from build123d import *

# Parameters (mm, degrees)
SKETCH_1_W      = 20
SKETCH_1_H      = 40
SKETCH_1_R      = 1.8
SKETCH_1_W_2    = 40
SKETCH_1_H_2    = 20
EXTRUDE_1_DEPTH = 3
FILLET_1_R      = 3


with BuildPart() as part:
    # 草图1 → 凸台-拉伸1 (new body)
    # profile 1 of 2: a face of its own
    with BuildSketch(Plane(origin=(0, 0, 0), x_dir=(1, 0, 0), z_dir=(0, 1, 0))):
        with Locations((-10, 30)):
            Rectangle(SKETCH_1_W, SKETCH_1_H)
        with Locations(Location((-10, 20, 0), (0, 0, 270))):
            Circle(SKETCH_1_R, mode=Mode.SUBTRACT)
        with Locations(Location((-10, 40, 0), (0, 0, 270))):
            Circle(SKETCH_1_R, mode=Mode.SUBTRACT)
    # profile 2 of 2: a face of its own
    with BuildSketch(Plane(origin=(0, 0, 0), x_dir=(1, 0, 0), z_dir=(0, 1, 0))):
        Rectangle(SKETCH_1_W_2, SKETCH_1_H_2)
        with Locations(Location((10, 0, 0), (0, 0, 270))):
            Circle(SKETCH_1_R, mode=Mode.SUBTRACT)
        with Locations(Location((-10, 0, 0), (0, 0, 270))):
            Circle(SKETCH_1_R, mode=Mode.SUBTRACT)
    extrude(amount=EXTRUDE_1_DEPTH)

    # 圆角1
    fillet_1_edges = [part.edges().sort_by_distance(p)[0] for p in [
        (-20, 1.5, -50),
        (0, 1.5, -50),
        (20, 1.5, -10),
        (20, 1.5, 10),
        (-20, 1.5, 10),
    ]]
    fillet(fillet_1_edges, radius=FILLET_1_R)


solid = part.part
Verification items for the finished model (mm, model axes). A direction names the side the tool comes from. Coordinates: 2 decimals unless noted, no trailing zeros. Order: outer loops, then holes, each group sorted by start corner. A loop starts at its lowest first (then second) coordinate and runs counter-clockwise, first axis right, second up. Notation, with made-up numbers: (87.5, 60) -> (125.5, 60) arc R22 ccw to (125.5, 70) -> close; hole circle Ø3 at (25, 20). An arc over 180 degrees is marked (long way). Put each result on its own line as item: value. Start each with the question number.
1. Cross-section at A-A, the plane z = -20. Record the boundary of the cut face in (x, y), then the cut area to 3 significant figures.
2. Cross-section at B-B, the plane x = 10. Record the boundary of the cut face in (y, z).
3. Cross-section at D-D, the plane x = -10. Record the boundary of the cut face in (y, z).
4. Access from +Z, -Z, +X, -X, +Y, -Y to the whole of each face (thin tool, end or side, straight path). Record for faces 4 (the flat face through (0, 1, -28)), 5 (the cylindrical face through (-11.597, 1.479, -39.169)).
5. Material ranges on L1, parallel to X at y = 1.9, z = 0; L2, parallel to X at y = 2.5, z = 0.5; L3, parallel to X at y = 2.3, z = -45, recorded low to high. Write a range as [from, to].
6. Go/stop test with flat-tipped pins: pin 1 Ø10 at (x, z) = (0, -8) entering from -Y; pin 2 Ø0.9 at (x, y) = (10.5, 1) entering from -Z. Record where each tip stops, or that it passes through.
7. Cross-section at C-C, the plane z = 0. Record the boundary of the cut face in (x, y), then the cut area to 3 significant figures.
8. Mould release check, pull along X, two halves, no side actions. Record for faces 1 (the cylindrical face through (8.243, 1.479, -0.39)), 2 (the cylindrical face through (-19.14, 1.52, -49.1)), 3 (the flat face through (-5, 3, -14)): released by +X, released by -X, zero draft, split by the parting line, or undercut.
Computed:
1. outline: (-20, 0) -> (-11.8, 0) -> (-11.8, 3) -> (-20, 3) -> close; (-8.2, 0) -> (0, 0) -> (0, 3) -> (-8.2, 3) -> close
1. area: 49.2 mm2
2. outline: (0, -10) -> (3, -10) -> (3, -1.8) -> (0, -1.8) -> close; (0, 1.8) -> (3, 1.8) -> (3, 10) -> (0, 10) -> close
3. outline: (0, -50) -> (3, -50) -> (3, -41.8) -> (0, -41.8) -> close; (0, -38.2) -> (3, -38.2) -> (3, -21.8) -> (0, -21.8) -> close; (0, -18.2) -> (3, -18.2) -> (3, -1.8) -> (0, -1.8) -> close; (0, 1.8) -> (3, 1.8) -> (3, 10) -> (0, 10) -> close
4. face 4: -Z, +X, +Y, -Y
4. face 5: +Y, -Y
5. L1: [-20, -11.8], [-8.2, 8.2], [11.8, 20]
5. L2: [-20, -11.73], [-8.27, 8.27], [11.73, 20]
5. L3: [-20, 0]
6. pin 1: y = 0
6. pin 2: z = -10
7. outline: (-20, 0) -> (-11.8, 0) -> (-11.8, 3) -> (-20, 3) -> close; (-8.2, 0) -> (8.2, 0) -> (8.2, 3) -> (-8.2, 3) -> close; (11.8, 0) -> (20, 0) -> (20, 3) -> (11.8, 3) -> close
7. area: 98.4 mm2
8. face 1: undercut
8. face 2: released by -X
8. face 3: zero draft
